Part model, mm, in its own coordinate system. A direction names the side the tool comes from. Round coordinates to 2 decimals unless told otherwise and drop trailing zeros. Write each loop counter-clockwise with the first axis right and the second up, starting at its lowest first coordinate (ties: lowest second). Pieces come first, ordered by that corner, then holes. Notation, with made-up numbers: (-23.75, 84.25) -> (-11.75, 84.25) arc R11 cw to (-11.75, 100.25) -> close; hole circle Ø10 at (6, -33.75). An arc over 180 degrees is marked (long way). Use CSV: the item, a comma, the result in double quotes. Start each with the question number.
(1) Which spindle directions (+Z, -Z, +X, -X, +Y, -Y) get a long thin tool onto all of the face, cutting with end or side? Do faces 1 (the flat face through (35, 22, 4)), 2 (the flat face through (-4, 22, 4)), 3 (the flat face through (33, 26.45, 2)), 4 (the flat face through (33, 17.45, 2)), 5 (the flat face through (2, 22, 1)). Say none if no direction does.
(2) Saw through at B-B (z = 0.7). Give the cut face in (x, y).
(3) Two-plate mould, pull along Y, no slides. Class faces 6 (the flat face through (-2, 17.45, 2)), 7 (the flat face through (15, 41.9, 1)), 8 (the flat face through (-2, 26.45, 2)): released by +Y, released by -Y, zero draft, split by the parting line, or undercut.
(4) Saw through at D-D (x = 6). Give the cut face in (y, z), plus the area to 3 significant figures.
(5) Drop flat-ended pins along their axis: pin 1 (2 mm diameter, centred on y = 15, z = 2, fed in from +X); pin 2 (3.5 mm diameter, centred on x = 33, y = 20.5, fed in from +Z); pin 3 (1.6 mm diameter, centred on x = 33, z = 1, fed in from -Y). Give the stop position or say it passes through.
(6) Saw through at C-C (x = 25.5). Give the cut face in (y, z).
(7) Probe line 1 (Y direction, x = 26, z = 1.5); line 2 (X direction, y = 24, z = 1.1); line 3 (Y direction, x = 25.5, z = 3.9). List the from-to ranges inside material, lowest first. Write a range as [from, to].
(8) Saw through at A-A (y = 9.5). Give the cut face in (x, z), plus the area to 3 significant figures.
```python
from build123d import *

# Parameters (mm, degrees)
SKETCH1_W           = 30.9
SKETCH1_H           = 43.9
SKETCH1_W_2         = 26.9
SKETCH1_H_2         = 39.9
BOSS_EXTRUDE1_DEPTH = 5
SKETCH2_W           = 30.9
SKETCH2_H           = 43.9
BOSS_EXTRUDE2_DEPTH = 2
BOSS_EXTRUDE3_DEPTH = 4
SKETCH4_R           = 4
CUT_EXTRUDE1_DEPTH  = 2
CUT_EXTRUDE2_DEPTH  = 60.199408781
FILLET1_R           = 3
FILLET2_R           = 0.8
SKETCH6_R           = 2.25
CUT_EXTRUDE3_DEPTH  = 60.199408781


with BuildPart() as part:
    # Sketch1 → Boss-Extrude1 (new body)
    with BuildSketch(Plane.XY):
        with Locations((15.45, 21.95)):
            Rectangle(SKETCH1_W, SKETCH1_H)
        with Locations((15.45, 21.95)):
            Rectangle(SKETCH1_W_2, SKETCH1_H_2, mode=Mode.SUBTRACT)
    extrude(amount=BOSS_EXTRUDE1_DEPTH)

    # Sketch2 → Boss-Extrude2 (add)
    with BuildSketch(Plane.XY.offset(5)):
        with Locations((15.45, 21.95)):
            Rectangle(SKETCH2_W, SKETCH2_H)
    extrude(amount=-BOSS_EXTRUDE2_DEPTH)

    # Sketch3 → Boss-Extrude3 (add)
    with BuildSketch(Plane(origin=(0, 0, 0), x_dir=(-1, 0, 0), z_dir=(0, 0, -1))):
        with BuildLine():
            Line((-34.9, 26.45), (-30.9, 26.45))
            Line((-30.9, 26.45), (-30.9, 17.45))
            Line((-30.9, 17.45), (-34.9, 17.45))
            ThreePointArc((-34.9, 17.45), (-39.4, 21.95), (-34.9, 26.45))
        make_face()
    boss_extrude3 = extrude(amount=-BOSS_EXTRUDE3_DEPTH)

    # Sketch4 → Cut-Extrude1 (cut)
    with BuildSketch(Plane(origin=(0, 0, 0), x_dir=(-1, 0, 0), z_dir=(0, 0, -1))):
        with Locations((-34.9, 21.95)):
            Circle(SKETCH4_R)
    cut_extrude1 = extrude(amount=-CUT_EXTRUDE1_DEPTH, mode=Mode.SUBTRACT)

    # Mirror1: Boss-Extrude3, Cut-Extrude1 across plane
    add(boss_extrude3.mirror(Plane(origin=(15.45, 0, 0), x_dir=(0, 0, 1), z_dir=(1, 0, 0))))
    add(cut_extrude1.mirror(Plane(origin=(15.45, 0, 0), x_dir=(0, 0, 1), z_dir=(1, 0, 0))), mode=Mode.SUBTRACT)

    # Sketch5 → Cut-Extrude2 (cut, through all)
    with BuildSketch(Plane.XY.offset(5)):
        with BuildLine():
            ThreePointArc((20.95, 29.9), (19.339087297, 33.789087297), (15.45, 35.4))
            Line((15.45, 35.4), (15.45, 24.4))
            ThreePointArc((15.45, 24.4), (19.339087297, 26.010912703), (20.95, 29.9))
        make_face()
        with BuildLine():
            Line((15.45, 24.4), (15.45, 35.4))
            ThreePointArc((15.45, 35.4), (9.95, 29.9), (15.45, 24.4))
        make_face()
    extrude(amount=-CUT_EXTRUDE2_DEPTH, mode=Mode.SUBTRACT)

    # Fillet1
    fillet1_edges = [part.edges().sort_by_distance(p)[0] for p in [
        (0, 0, 2.5),
        (0, 43.9, 2.5),
        (30.9, 43.9, 2.5),
        (30.9, 0, 2.5),
    ]]
    fillet(fillet1_edges, radius=FILLET1_R)

    # Fillet2
    fillet2_edges = [part.edges().sort_by_distance(p)[0] for p in [
        (15.45, 0, 5),
        (15.45, 43.9, 5),
        (0, 21.95, 5),
        (0.878679656, 43.021320344, 5),
        (30.021320344, 43.021320344, 5),
        (0.878679656, 0.878679656, 5),
        (30.021320344, 0.878679656, 5),
        (39.4, 21.95, 4),
        (32.9, 26.45, 4),
        (32.9, 17.45, 4),
        (-8.5, 21.95, 4),
        (-2, 17.45, 4),
        (-2, 26.45, 4),
        (15.45, 35.4, 5),
        (30.9, 21.95, 5),
    ]]
    fillet(fillet2_edges, radius=FILLET2_R)

    # Sketch6 → Cut-Extrude3 (cut, through all)
    with BuildSketch(Plane.XY.offset(5)):
        with Locations((25.5, 9.5)):
            Circle(SKETCH6_R)
    extrude(amount=-CUT_EXTRUDE3_DEPTH, mode=Mode.SUBTRACT)


solid = part.part
```
Answers:
1,face 1,"+Z, +X, +Y, -Y"
1,face 2,"+Z, -X, +Y, -Y"
1,face 3,"+Z, -Z, +X, +Y"
1,face 4,"+Z, -Z, +X, -Y"
1,face 5,"-Z"
2,outline,"(-4, 17.45) -> (0, 17.45) -> (0, 3) arc R3 ccw to (3, 0) -> (27.9, 0) arc R3 ccw to (30.9, 3) -> (30.9, 17.45) -> (34.9, 17.45) arc R4.5 ccw to (34.9, 26.45) -> (30.9, 26.45) -> (30.9, 40.9) arc R3 ccw to (27.9, 43.9) -> (3, 43.9) arc R3 ccw to (0, 40.9) -> (0, 26.45) -> (-4, 26.45) arc R4.5 ccw to start; hole circle Ø8 at (-4, 21.95); hole (2, 2) -> (28.9, 2) -> (28.9, 41.9) -> (2, 41.9) -> close; hole circle Ø8 at (34.9, 21.95)"
3,face 6,"released by -Y"
3,face 7,"undercut"
3,face 8,"released by +Y"
4,outline,"(0, 0) -> (2, 0) -> (2, 3) -> (41.9, 3) -> (41.9, 0) -> (43.9, 0) -> (43.9, 4.2) arc R0.8 ccw to (43.1, 5) -> (0.8, 5) arc R0.8 ccw to (0, 4.2) -> close"
4,area,"99.5 mm²"
5,pin 1,"stops at x = 30.9"
5,pin 2,"stops at z = 4"
5,pin 3,"stops at y = 17.45"
6,outline,"(0, 0) -> (2, 0) -> (2, 3) -> (7.25, 3) -> (7.25, 5) -> (0.8, 5) arc R0.8 ccw to (0, 4.2) -> close; (11.75, 3) -> (41.9, 3) -> (41.9, 0) -> (43.9, 0) -> (43.9, 4.2) arc R0.8 ccw to (43.1, 5) -> (11.75, 5) -> close"
7,line 1,"y = [0, 2], [41.9, 43.9]"
7,line 2,"x = [-8.01, -7.43], [-0.57, 2], [28.9, 31.47], [38.33, 38.91]"
7,line 3,"y = [0, 7.25], [11.75, 43.9]"
8,outline,"(0, 0) -> (2, 0) -> (2, 3) -> (23.25, 3) -> (23.25, 5) -> (0.8, 5) arc R0.8 ccw to (0, 4.2) -> close; (27.75, 3) -> (28.9, 3) -> (28.9, 0) -> (30.9, 0) -> (30.9, 4.2) arc R0.8 ccw to (30.1, 5) -> (27.75, 5) -> close"
8,area,"64.5 mm²"
